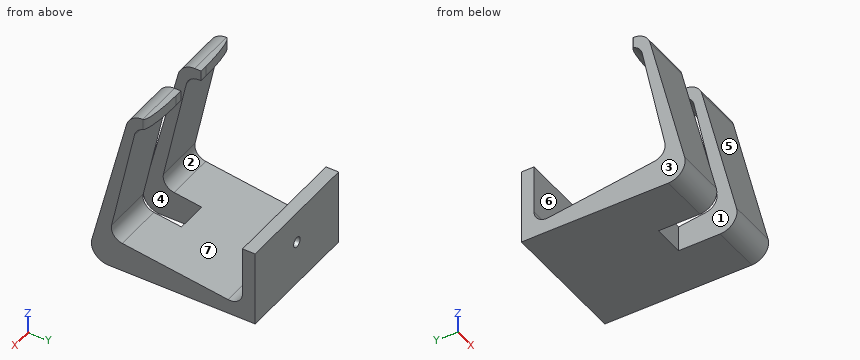
```python
from build123d import *

# Parameters (mm, degrees)
BOSS_EXTRUDE1_DEPTH                                 = 31
FILLET1_SIZE                                        = 20
FILLET1_SIZE_2                                      = 3
FILLET2_SIZE                                        = 3
FILLET2_SIZE_2                                      = 20
CUT_EXTRUDE1_DEPTH                                  = 91.700411417
CUT_EXTRUDE1_DEPTH_BACK                             = 91.700411417
SKETCH2_W                                           = 15
SKETCH2_H                                           = 30
CSK_FOR_M4_COUNTERSUNK_FLAT_HEAD_SCREW1_D           = 4.8
CSK_FOR_M4_COUNTERSUNK_FLAT_HEAD_SCREW1_DEPTH       = 15.2
CSK_FOR_M4_COUNTERSUNK_FLAT_HEAD_SCREW1_CSINK_D     = 9.4
CSK_FOR_M4_COUNTERSUNK_FLAT_HEAD_SCREW1_CSINK_ANGLE = 90
CSK_FOR_M4_COUNTERSUNK_FLAT_HEAD_SCREW1_TIP         = 1.442065486


with BuildPart() as part:
    # Sketch1 → Boss-Extrude1 (new, symmetric)
    with BuildSketch(Plane(origin=(0, 0, 0), x_dir=(0, 0, -1), z_dir=(1, 0, 0))):
        with BuildLine():
            Line((0, 0), (23.097789557, 0))
            ThreePointArc((23.097789557, 0), (27.626047038, -2.063645826), (29.039397969, -6.835038606))
            Line((29.039397969, -6.835038606), (21.973887052, -57.10876106))
            ThreePointArc((21.973887052, -57.10876106), (19.473737257, -61.18863472), (14.784808494, -62.142608059))
            Line((14.784808494, -62.142608059), (-36.247470145, -51.295362377))
            ThreePointArc((-36.247470145, -51.295362377), (-39.662875769, -49.202399119), (-41, -45.426476772))
            Line((-41, -45.426476772), (-41, -44.285180972))
            Line((-41, -44.285180972), (-46, -44.285180972))
            Line((-46, -44.285180972), (-46, -47.304818755))
            ThreePointArc((-46, -47.304818755), (-44.304086029, -52.230110557), (-39.935375165, -55.067184565))
            Line((-39.935375165, -55.067184565), (26.064624835, -71.522832753))
            ThreePointArc((26.064624835, -71.522832753), (32.925291803, -70.064552971), (36, -63.760466942))
            Line((36, -63.760466942), (36, 6))
            Line((36, 6), (0, 6))
            Line((0, 6), (0, 0))
        make_face()
    extrude(amount=BOSS_EXTRUDE1_DEPTH, both=True)

    # Fillet1
    # an asymmetric fillet: 20, 3 mm, written as the material it takes off along each edge
    with BuildSketch(Plane(origin=(-31, -44.285180972, -9), x_dir=(1, 0, 0), z_dir=(0, 0, 1))) as fillet1_piece_1:
        with BuildLine():
            Bezier((FILLET1_SIZE, 0), (0, 0), (0, -FILLET1_SIZE_2), weights=[1, 0.707106781, 1])
            Line((0, -FILLET1_SIZE_2), (0, 0))
            Line((0, 0), (FILLET1_SIZE, 0))
        make_face()
    extrude(amount=105, mode=Mode.SUBTRACT)

    # Fillet2
    # an asymmetric fillet: 20, 3 mm, written as the material it takes off along each edge
    with BuildSketch(Plane(origin=(31, -44.285180972, -9), x_dir=(0, -1, 0), z_dir=(0, 0, 1))) as fillet2_piece_1:
        with BuildLine():
            Bezier((FILLET2_SIZE, 0), (0, 0), (0, -FILLET2_SIZE_2), weights=[1, 0.707106781, 1])
            Line((0, -FILLET2_SIZE_2), (0, 0))
            Line((0, 0), (FILLET2_SIZE, 0))
        make_face()
    extrude(amount=105, mode=Mode.SUBTRACT)

    # Sketch2 → Cut-Extrude1 (cut, two sides: drawn at the far end of the back side and taken through both)
    with BuildSketch(Plane.XY.offset(-CUT_EXTRUDE1_DEPTH_BACK)):
        with Locations((0, -59)):
            Rectangle(SKETCH2_W, SKETCH2_H)
    extrude(amount=CUT_EXTRUDE1_DEPTH + CUT_EXTRUDE1_DEPTH_BACK, mode=Mode.SUBTRACT)

    # CSK for M4 Countersunk Flat Head Screw1
    with Locations(Plane(origin=(0, 0, -15), x_dir=(0, 0, -1), z_dir=(0, -1, 0))):
        with Locations((0, 0)):
            CounterSinkHole(CSK_FOR_M4_COUNTERSUNK_FLAT_HEAD_SCREW1_D / 2, CSK_FOR_M4_COUNTERSUNK_FLAT_HEAD_SCREW1_CSINK_D / 2, depth=CSK_FOR_M4_COUNTERSUNK_FLAT_HEAD_SCREW1_DEPTH, counter_sink_angle=CSK_FOR_M4_COUNTERSUNK_FLAT_HEAD_SCREW1_CSINK_ANGLE)
            with Locations((0, 0, -(CSK_FOR_M4_COUNTERSUNK_FLAT_HEAD_SCREW1_DEPTH + CSK_FOR_M4_COUNTERSUNK_FLAT_HEAD_SCREW1_TIP / 2))):  # 118° drill point
                Cone(0, CSK_FOR_M4_COUNTERSUNK_FLAT_HEAD_SCREW1_D / 2, CSK_FOR_M4_COUNTERSUNK_FLAT_HEAD_SCREW1_TIP, mode=Mode.SUBTRACT)


solid = part.part
```
Can you work these out from the model? Positions are in its coordinate system, mm. Face numbers are marked on the shaded views. A direction names the side the tool comes from. Round coordinates to 2 decimals unless told otherwise and drop trailing zeros. Order: outer loops, then holes, each group sorted by start corner. A loop starts at its lowest first (then second) coordinate and runs counter-clockwise, first axis right, second up. Notation, with made-up numbers: (-11, 16.25) -> (16, 16.25) arc R25 ccw to (16, 45.25) -> close; hole circle Ø6 at (-13.75, 20.25). An arc over 180 degrees is marked (long way). Return JSON: item names as keys, results as strings. Group by question number.
1. We'd pull the mould along Y, two halves only. Please class the marked faces 4, 5, 6 and 7: released by +Y, released by -Y, zero draft, split by the parting line, or undercut.
2. If we section it at C-C, the plane y = -66.5: Write out the boundary of the cut face in (x, z).
3. Which directions (+Z, -Z, +X, -X, +Y, -Y) give clear straight access to the entire face, cutting with the end or side of a thin tool? Please do the marked faces 1, 2 and 3.
4. If we section it at A-A, the plane x = 0: Write out the boundary of the cut face in (y, z), then the cut area to 3 significant figures.
5. I need wall thicknesses on line 1 (X direction, y = 5, z = -15); line 2 (Z direction, x = 0, y = 3.35); line 3 (X direction, y = -64, z = -25.5). Which ranges of each line are inside material? Lowest first, please. Write a range as [from, to].
6. Will these pins go through, and if not, where does the flat tip stop? pin 1 (22 mm diameter, centred on y = -52.5, z = -11, fed in from +X); pin 2 (10 mm diameter, centred on x = -7.5, z = 9.5, fed in from -Y); pin 3 (4 mm diameter, centred on x = 19, z = 29, fed in from +Y); pin 4 (4.5 mm diameter, centred on x = 0, z = -15, fed in from -Y).
7. If we section it at D-D, the plane y = -54: Write out the boundary of the cut face in (x, z).
8. If we section it at B-B, the plane z = 18: Write out the boundary of the cut face in (x, y).
Output values:
{
 "1": {"face 4": "zero draft", "face 5": "released by -Y", "face 6": "undercut", "face 7": "undercut"},
 "2": {"outline": "(-31, -35.52) -> (-7.5, -35.52) -> (-7.5, -5.92) -> (-31, -5.92) -> close; (7.5, -35.52) -> (31, -35.52) -> (31, -5.92) -> (7.5, -5.92) -> close"},
 "3": {"face 1": "+Z, -Z, -Y", "face 2": "+X, -X", "face 3": "+Z, -Z, -X, +Y, -Y"},
 "4": {"outline": "(-44, -36) -> (6, -36) -> (6, -17.4) -> (2.3, -17.4) -> (0, -19.7) -> (0, -23.1) arc R6 cw to (-6.84, -29.04) -> (-44, -23.82) -> close; (0, -10.3) -> (2.3, -12.6) -> (6, -12.6) -> (6, 0) -> (0, 0) -> close", "area": "593 mm²"},
 "5": {"line 1": "[-31, -2.4], [2.4, 31]", "line 2": "[-36, -17.4], [-12.6, 0]", "line 3": "[-31, -7.5], [7.5, 31]"},
 "6": {"pin 1": "x = 31", "pin 2": "y = -63.9", "pin 3": "y = -52.41", "pin 4": "through"},
 "7": {"outline": "(-31, -36) -> (-7.5, -36) -> (-7.5, -22.41) -> (-31, -22.41) -> close; (-31, 23.52) -> (-7.5, 23.52) -> (-7.5, 42.38) -> (-31, 42.38) -> close; (7.5, -36) -> (31, -36) -> (31, -22.41) -> (7.5, -22.41) -> close; (7.5, 23.52) -> (31, 23.52) -> (31, 42.38) -> (7.5, 42.38) -> close"},
 "8": {"outline": "(-31, -60.54) -> (-7.5, -60.54) -> (-7.5, -55.17) -> (-31, -55.17) -> close; (7.5, -60.54) -> (31, -60.54) -> (31, -55.17) -> (7.5, -55.17) -> close"}
}
